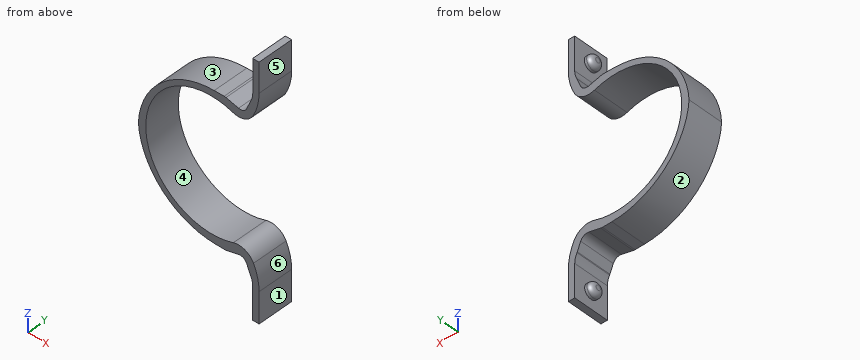
```python
from build123d import *

# Parameters (mm, degrees)
BOSS_EXTRUDE1_DEPTH = 15
FILLET1_R           = 33
FILLET3_R           = 8
SKETCH3_W           = 14.976754218
SKETCH3_H           = 50.502927364
CUT_EXTRUDE1_DEPTH  = 71.805882398
FILLET4_R           = 13
FILLET5_R           = 23
CUT_EXTRUDE2_DEPTH  = 71.805882398
FILLET6_R           = 3
FILLET7_R           = 7
SKETCH11_R          = 2.99322587
BOSS_EXTRUDE3_DEPTH = 3
SKETCH12_R          = 3.00628595
BOSS_EXTRUDE4_DEPTH = 3
FILLET15_R          = 2


with BuildPart() as part:
    # Sketch1 → Boss-Extrude1 (new body)
    with BuildSketch(Plane(origin=(0, 0, 0), x_dir=(1, 0, 0), z_dir=(0, 1, 0))):
        with BuildLine():
            Line((13.49710544, 37.52594122), (-35.345435735, 37.52594122))
            Line((-35.345435735, 37.52594122), (-35.345435735, -23.95909877))
            Line((-35.345435735, -23.95909877), (13.519906977, -24.812641875))
            Line((13.519906977, -24.812641875), (13.519906977, -46.812641875))
            Line((13.519906977, -46.812641875), (16.216594819, -46.812641875))
            Line((16.216594819, -46.812641875), (16.216594819, -12.903441484))
            ThreePointArc((16.216594819, -12.903441484), (-32.140827884, 6.320900922), (16.216594819, 25.545243327))
            Line((16.216594819, 25.545243327), (16.216594819, 59.52594122))
            Line((16.216594819, 59.52594122), (13.49710544, 59.52594122))
            Line((13.49710544, 59.52594122), (13.49710544, 37.52594122))
        make_face()
    extrude(amount=BOSS_EXTRUDE1_DEPTH)

    # Fillet1
    # the kernel refuses this fillet: 33 mm, written as the material it takes off along each edge
    with BuildSketch(Plane(origin=(-35.345435735, -81.071536578, 23.95909877), x_dir=(0, 0, -1), z_dir=(0, 1, 0))) as fillet1_piece_1:
        with BuildLine():
            CenterArc((FILLET1_R * 0.98268529185, -FILLET1_R), FILLET1_R, 90, 88.999302122)
            Line((-FILLET1_R * 0.0171621906577, -FILLET1_R * 0.982535415153), (0, 0))
            Line((0, 0), (FILLET1_R * 0.98268529185, 0))
        make_face()
    extrude(amount=177.143073155, mode=Mode.SUBTRACT)
    with BuildSketch(Plane(origin=(-35.345435735, -82.5, -37.52594122), x_dir=(1, 0, 0), z_dir=(0, 1, 0))) as fillet1_piece_2:
        with BuildLine():
            CenterArc((FILLET1_R, -FILLET1_R), FILLET1_R, 90, 90)
            Line((0, -FILLET1_R), (0, 0))
            Line((0, 0), (FILLET1_R, 0))
        make_face()
    extrude(amount=180, mode=Mode.SUBTRACT)

    # Fillet3
    fillet3_edges = [part.edges().sort_by_distance(p)[0] for p in [
        (13.519906977, 7.5, 24.812641875),
        (13.49710544, 7.5, -37.52594122),
    ]]
    fillet(fillet3_edges, radius=FILLET3_R)

    # Sketch3 → Cut-Extrude1 (cut, through all)
    with BuildSketch(Plane(origin=(0, 15, 0), x_dir=(1, 0, 0), z_dir=(0, 1, 0))):
        with Locations((13.189850954, 6.26949409)):
            Rectangle(SKETCH3_W, SKETCH3_H)
    extrude(amount=-CUT_EXTRUDE1_DEPTH, mode=Mode.SUBTRACT)

    # Fillet4
    fillet4_edges = [part.edges().sort_by_distance(p)[0] for p in [
        (8.063971776, 7.5, -31.520957772),
        (7.849365767, 7.5, 18.981969592),
    ]]
    fillet(fillet4_edges, radius=FILLET4_R)

    # Fillet5
    # the kernel refuses this fillet: 23 mm, written as the material it takes off along each edge
    with BuildSketch(Plane(origin=(16.216594819, -37.21201477, -31.520957772), x_dir=(-1, 0, 0), z_dir=(0, 1, 0))) as fillet5_piece_1:
        with BuildLine():
            CenterArc((23, -14.884805908), FILLET5_R, 139.671769874, 40.328230126)
            Line((0, -14.884805908), (-0.46, -14.884805908))
            Line((-0.46, -14.884805908), (-0.46, 0))
            Line((-0.46, 0), (0, 0.46))
            ThreePointArc((0, 0.46), (2.73298008, 0.46), (5.115279364, 0.297696118))
            Line((5.115279364, 0.297696118), (5.465960161, 0))
        make_face()
    extrude(amount=89.424029541, mode=Mode.SUBTRACT)
    with BuildSketch(Plane(origin=(16.216594819, 52.982840025, 18.981969592), x_dir=(-1, 0, 0), z_dir=(0, -1, 0))) as fillet5_piece_2:
        with BuildLine():
            CenterArc((23, -15.19313601), FILLET5_R, 138.656554967, 41.343445033)
            Line((0, -15.19313601), (-0.46, -15.19313601))
            Line((-0.46, -15.19313601), (-0.46, 0))
            Line((-0.46, 0), (0, 0.46))
            ThreePointArc((0, 0.46), (2.866220147, 0.46), (5.3870891, 0.30386272))
            Line((5.3870891, 0.30386272), (5.732440294, 0))
        make_face()
    extrude(amount=90.96568005, mode=Mode.SUBTRACT)

    # Sketch4 → Cut-Extrude2 (cut, through all)
    with BuildSketch(Plane(origin=(0, 15, 0), x_dir=(1, 0, 0), z_dir=(0, 1, 0))):
        Polygon((1.715705502, -24.606454949), (9.959521951, -22.566105124), (13.119950571, -30.176257645), align=None)
        Polygon((13.119950571, 43.171714726), (1.715705502, 37.60191203), (9.959521951, 35.561562205), align=None)
    extrude(amount=-CUT_EXTRUDE2_DEPTH, mode=Mode.SUBTRACT)

    # Fillet6
    # the kernel refuses this fillet: 3 mm, written as the material it adds along each edge
    with BuildSketch(Plane(origin=(9.959521951, 15, 22.566105124), x_dir=(0.38353267260391577, 0, 0.9235273082293222), z_dir=(0, -1, 0)), Plane(origin=(9.959521951, 15, -35.561562205), x_dir=(-0.9707106735613967, 0, -0.24025151036773845), z_dir=(0, -1, 0))) as fillet6_piece_1:
        with BuildLine():
            CenterArc((FILLET6_R * 0.859357235827, FILLET6_R), FILLET6_R, 188.651291771, 81.348708229)
            Line((-FILLET6_R * 0.129264883466, FILLET6_R * 0.849579571712), (0, 0))
            Line((0, 0), (FILLET6_R * 0.859357235827, 0))
        make_face()
    extrude(amount=15)
    # the kernel refuses this fillet: 3 mm, written as the material it takes off along each edge
    with BuildSketch(Plane(origin=(12.653561764, -0.262717319, 29.053216951), x_dir=(-0.3835326726039229, 0, -0.9235273082293193), z_dir=(0, 1, 0))) as fillet6_2_piece_1:
        with BuildLine():
            CenterArc((0.105086928, -3), FILLET6_R, 90, 3.716956431)
            ThreePointArc((-0.089395975, -0.00631057), (-0.044689151, -0.003280466), (0, 0))
            Line((0, 0), (0.105086928, 0))
        make_face()
    extrude(amount=15.525434639, mode=Mode.SUBTRACT)
    with BuildSketch(Plane(origin=(12.466360821, -0.41333627, -41.597903613), x_dir=(0.4833086879383824, 0, -0.8754500055190354), z_dir=(0, 1, 0))) as fillet6_2_piece_2:
        with BuildLine():
            CenterArc((0.167434819, -2.999883511), FILLET6_R, 90.504917507, 5.844127099)
            Line((-0.164320455, -0.018283532), (0, 0))
            ThreePointArc((0, 0), (0.070498871, -0.000310637), (0.140997742, 0))
        make_face()
    extrude(amount=15.826672539, mode=Mode.SUBTRACT)
    with BuildSketch(Plane(origin=(1.715705502, 15.980874738, 24.606454949), x_dir=(-0.9998474825072629, 0, -0.017464584847299507), z_dir=(0, -1, 0))) as fillet6_2_piece_3:
        with BuildLine():
            CenterArc((FILLET6_R * 0.130783298337, FILLET6_R), FILLET6_R, 255.097916944, 14.902083056)
            Line((-FILLET6_R * 0.126384628394, FILLET6_R * 0.0336332696842), (0, 0))
            Line((0, 0), (FILLET6_R * 0.130783298337, 0))
        make_face()
    extrude(amount=16.961749475, mode=Mode.SUBTRACT)
    with BuildSketch(Plane(origin=(2.022657479, 15.914333267, -37.52594122), x_dir=(0.9707106735613966, 0, 0.24025151036773865), z_dir=(0, -1, 0))) as fillet6_2_piece_4:
        with BuildLine():
            CenterArc((FILLET6_R * 0.121911102219, FILLET6_R), FILLET6_R, 256.098614822, 13.901385178)
            Line((-FILLET6_R * 0.118340408149, FILLET6_R * 0.0292893264386), (0, 0))
            Line((0, 0), (FILLET6_R * 0.121911102219, 0))
        make_face()
    extrude(amount=16.828666533, mode=Mode.SUBTRACT)

    # Fillet7
    fillet7_edges = [part.edges().sort_by_distance(p)[0] for p in [
        (10.484154524, 7.5, 18.981969592),
        (10.750634658, 7.5, -31.520957772),
    ]]
    fillet(fillet7_edges, radius=FILLET7_R)

    # Sketch11 → Boss-Extrude3 (add)
    with BuildSketch(Plane.ZY.offset(-13.519906977)):
        with Locations((39.731607941, 7.574163162)):
            Circle(SKETCH11_R)
    extrude(amount=BOSS_EXTRUDE3_DEPTH)

    # Sketch12 → Boss-Extrude4 (add)
    with BuildSketch(Plane.ZY.offset(-13.49710544)):
        with Locations((-52.589854429, 7.422107304)):
            Circle(SKETCH12_R)
    extrude(amount=BOSS_EXTRUDE4_DEPTH)

    # Fillet15
    fillet15_edges = [part.edges().sort_by_distance(p)[0] for p in [
        (10.519906977, 7.574163162, 36.738382071),
        (10.49710544, 7.422107304, -55.59614038),
    ]]
    fillet(fillet15_edges, radius=FILLET15_R)


solid = part.part
```
Verification items for the finished model (mm, model axes). Face numbers are marked on the shaded views. A direction names the side the tool comes from. Round coordinates to 2 decimals unless told otherwise and drop trailing zeros. Order: outer loops, then holes, each group sorted by start corner. A loop starts at its lowest first (then second) coordinate and runs counter-clockwise, first axis right, second up.
1) Cross-section at D-D, the plane z = -40. Record the cut outline in (x, y).
Geometry says:
outline: (11.8, 0) - (15.31, 0) - (15.31, 15) - (11.8, 15) - close
2) Draft check along Z on the marked faces 1, 2, 3 and 4. Enter one of: +Z half, -Z half, draft (parallel to the pull), parting line (faces both ways), or undercut.
Geometry says:
face 1: draft
face 2: -Z half
face 3: +Z half
face 4: undercut
3) Cross-section at C-C, the plane z = -12. Record the cut outline in (x, y).
Geometry says:
outline: (-34.49, 0) - (-31.56, 0) - (-31.56, 15) - (-34.49, 15) - close
4) Depth check by flat-ended pin: pin 1 (8 mm diameter, centred on y = 10.5, z = -37, fed in from -X); pin 2 (3 mm diameter, centred on x = -1.5, y = 8, fed in from -Z); pin 3 (3 mm diameter, centred on x = -2, y = 3.5, fed in from +Z). Enter the tip coordinate at first touch or a pass-through.
Geometry says:
pin 1: stops at x = -19.03
pin 2: stops at z = -37.53
pin 3: stops at z = 24.57
5) Cross-section at B-B, the plane x = -4.5. Record the cut outline in (y, z).
Geometry says:
outline: (0, -37.46) - (15, -37.46) - (15, -34.32) - (0, -34.32) - close; (0, 21.68) - (15, 21.68) - (15, 24.46) - (0, 24.46) - close
6) Material ranges on line 1 (Z direction, x = 11.5, y = 6.25); line 2 (X direction, y = 3, z = -46); line 3 (Z direction, x = -29, y = 3.5), recorded low to high.
Geometry says:
line 1: z = -55.07 to -50.11, -39.27 to -33.53, 21.07 to 26.28, 37.36 to 42.1
line 2: x = 13.5 to 16.21
line 3: z = -23.98 to -19.21, 6.56 to 10.99
7) Cross-section at A-A, the plane x = -13.5. Record the cut outline in (y, z), plus the area to 3 significant figures.
Geometry says:
outline: (0, -35.58) - (15, -35.58) - (15, -32.71) - (0, -32.71) - close; (0, 20.07) - (15, 20.07) - (15, 22.59) - (0, 22.59) - close
area: 80.9 mm2
8) Tool access check on the marked faces 5 and 6. Record the directions out of +Z, -Z, +X, -X, +Y, -Y that give a thin tool (end or side, any length) a straight path to the whole face; none if there is none.
Geometry says:
face 5: +Z, -Z, +X, +Y, -Y
face 6: +X, +Y, -Y
